Source: CAD feature listing. Evaluate the final solid. Frame: model axes, mm. Round coordinates to 2 decimals unless told otherwise and drop trailing zeros. Write each loop counter-clockwise with the first axis right and the second up, starting at its lowest first coordinate (ties: lowest second). Pieces come first, ordered by that corner, then holes. Notation, with made-up numbers: M 35.25,9 L 89.25,9 A24 cw 89.25,46 Z; hole C -15.5,2.25 d4. An arc over 180 degrees is marked long. Answer in a Markdown table with one row per item.
from build123d import *

# Parameters (mm, degrees)
F1_DEPTH = 20


with BuildPart() as f1:
    # F0 (on Top) → F1 (new body)
    with BuildSketch(Plane.XY):
        with BuildLine():
            Line((0, 602.120165), (-8.537433, 158.088193))
            Line((-8.537433, 158.088193), (-11.36, -19.861807))
            ThreePointArc((-11.36, -19.861807), (-9.968781, -23.757604), (-6.36, -25.779835))
            ThreePointArc((-6.36, -25.779835), (6.778319, -27.353029), (20, -27.879835))
            ThreePointArc((20, -27.879835), (33.221681, -27.353029), (46.36, -25.779835))
            ThreePointArc((46.36, -25.779835), (49.968781, -23.757604), (51.36, -19.861807))
            Line((51.36, -19.861807), (48.537433, 158.088193))
            Line((48.537433, 158.088193), (40, 602.120165))
            Line((40, 602.120165), (20, 602.120165))
            Line((20, 602.120165), (0, 602.120165))
        make_face()
    extrude(amount=F1_DEPTH)


solid = f1.part
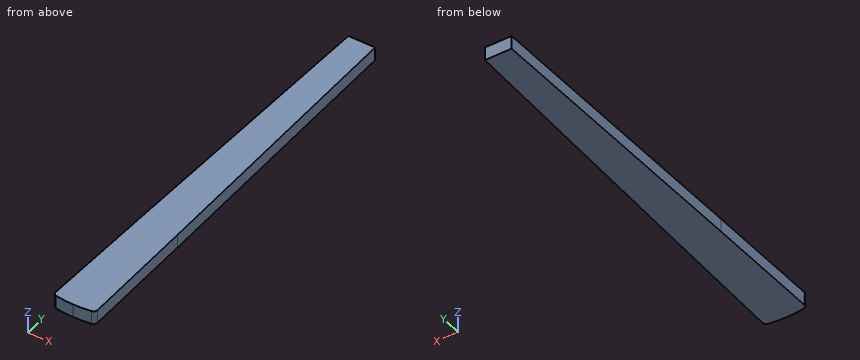
Q1. Section B-B (y = 207.5). Return loops of the section in (x, z), and give its area (3 significant figures).
Solutions:
| item | result |
|---|---|
| outline | M -7.59,0 L 47.59,0 L 47.59,20 L -7.59,20 Z |
| area | 1,100 mm2 |
Q2. Contact query for flat-ended pins moving along their axis: pin 1 Ø4 at (y, z) = (297, 2.5) entering from +X (3 decimals); pin 2 Ø1 at (y, z) = (292.5, 12.5) entering from -X; pin 3 Ø5 at (y, z) = (533.5, 13.5) entering from +X. Output: stop coordinate, or through.
Solutions:
| item | result |
|---|---|
| pin 1 | stops at x = 45.905 |
| pin 2 | stops at x = -5.96 |
| pin 3 | stops at x = 41.37 |
Q3. Material intervals for probe 1 along Y at (x, z) = (21.5, 11.5); probe 2 along Y at (x, z) = (14, 17.5); probe 3 along X at (y, z) = (360, 12.25), sorted ascending.
Solutions:
| item | result |
|---|---|
| probe 1 | y = -27.87 to 602.12 |
| probe 2 | y = -27.77 to 602.12 |
| probe 3 | x = -4.66 to 44.66 |
Q4. Section A-A (z = 7.5). Return loops of the section in (x, y), and give its area (3 significant figures).
Solutions:
| item | result |
|---|---|
| outline | M -11.36,-19.86 A5.89 ccw -6.36,-25.78 A166.8 ccw 20,-27.88 A166.8 ccw 46.36,-25.78 A5.89 ccw 51.36,-19.86 L 48.54,158.09 L 40,602.12 L 0,602.12 L -8.54,158.09 Z |
| area | 32,600 mm2 |
Q5. Section C-C (y = 88.5). Return loops of the section in (x, z).
Solutions:
| item | result |
|---|---|
| outline | M -9.64,0 L 49.64,0 L 49.64,20 L -9.64,20 Z |
